Read the model definition and answer for the solid it produces. Units are mm, in the model's axes. A direction names the side the tool comes from. Round coordinates to 2 decimals unless told otherwise and drop trailing zeros. Order: outer loops, then holes, each group sorted by start corner. A loop starts at its lowest first (then second) coordinate and runs counter-clockwise, first axis right, second up. Notation, with made-up numbers: (23.25, 66.5) -> (58.25, 66.5) arc R18 ccw to (58.25, 101.5) -> close; hole circle Ø4 at (49.5, -14). An arc over 180 degrees is marked (long way). Answer as a JSON object with one key per item and string values. Group by question number.
Item 1: Section C-C, the plane z = -9 is taken. Write down the section's boundary in (x, y), plus the area to 3 significant figures.
Item 2: For faces 1 (the cylindrical face through (22.15, 22.6, -13.87)), 2 (the flat face through (-1, 15, 8.899)), determine the directions among +Z, -Z, +X, -X, +Y, -Y from which every point of the face is accessible in a straight line to the end or side of a thin tool.
Item 3: The mould has two halves that part along X. Classify faces 3 (the flat face through (40, 15, -11)), 4 (the cylindrical face through (-22.15, 22.6, -8.33)), 5 (the flat face through (-1, 30, -11)): pulls with the +X half, pulls with the -X half, needs draft (parallel to the pull), parting line crosses it, or undercut.
Item 4: Section B-B, the plane y = 12.5 is taken. Write down the section's boundary in (x, z), plus the area to 3 significant figures.
Item 5: Section A-A, the plane x = -33 is taken. Write down the section's boundary in (y, z), plus the area to 3 significant figures.
Item 6: Consider probe 1 along X at (y, z) = (19.75, -13.5); probe 2 along X at (y, z) = (20.75, -8.5); probe 3 along Z at (x, y) = (-23, 28.25). Determine where each line is inside the solid, lowest interval first. Write a range as from..to.
Item 7: Section D-D, the plane y = 19 is taken. Write down the section's boundary in (x, z), plus the area to 3 significant figures.
from build123d import *

# Parameters (mm, degrees)
SKETCH1_W           = 80
SKETCH1_H           = 40
SKETCH1_R           = 3
BOSS_EXTRUDE1_DEPTH = 30
SKETCH2_R           = 3
CUT_EXTRUDE1_DEPTH  = 15


with BuildPart() as part:
    # Sketch1 → Boss-Extrude1 (new body)
    with BuildSketch(Plane(origin=(0, 0, 0), x_dir=(1, 0, 0), z_dir=(0, 1, 0))):
        with Locations((0, 11.100547393)):
            Rectangle(SKETCH1_W, SKETCH1_H)
        with Locations(Location((-33, 11.100547393, 0), (0, 0, 270))):  # turned: the seam where the file's is
            Circle(SKETCH1_R, mode=Mode.SUBTRACT)
        with Locations(Location((33, 11.100547393, 0), (0, 0, 90))):  # turned: the seam where the file's is
            Circle(SKETCH1_R, mode=Mode.SUBTRACT)
    extrude(amount=BOSS_EXTRUDE1_DEPTH)

    # Sketch2 → Cut-Extrude1 (cut)
    with BuildSketch(Plane(origin=(0, 30, 0), x_dir=(-1, 0, 0), z_dir=(0, 1, 0))):
        with Locations(Location((21, -11.100547393, 0), (0, 0, 90))):  # turned: the seam where the file's is
            Circle(SKETCH2_R)
        with Locations(Location((-21, -11.100547393, 0), (0, 0, 270))):  # turned: the seam where the file's is
            Circle(SKETCH2_R)
    extrude(amount=-CUT_EXTRUDE1_DEPTH, mode=Mode.SUBTRACT)


solid = part.part
Values found:
{
 "1": {"outline": "(-40, 0) -> (-35.14, 0) -> (-35.14, 30) -> (-40, 30) -> close; (-30.86, 0) -> (30.86, 0) -> (30.86, 30) -> (23.14, 30) -> (23.14, 15) -> (18.86, 15) -> (18.86, 30) -> (-18.86, 30) -> (-18.86, 15) -> (-23.14, 15) -> (-23.14, 30) -> (-30.86, 30) -> close; (35.14, 0) -> (40, 0) -> (40, 30) -> (35.14, 30) -> close", "area": "2,010 mm2"},
 "2": {"face 1": "+Y", "face 2": "+Z, +X, -X, +Y, -Y"},
 "3": {"face 3": "pulls with the +X half", "face 4": "undercut", "face 5": "needs draft"},
 "4": {"outline": "(-40, -31.1) -> (40, -31.1) -> (40, 8.9) -> (-40, 8.9) -> close; hole circle Ø6 at (-33, -11.1); hole circle Ø6 at (33, -11.1)", "area": "3,140 mm2"},
 "5": {"outline": "(0, -31.1) -> (30, -31.1) -> (30, -14.1) -> (0, -14.1) -> close; (0, -8.1) -> (30, -8.1) -> (30, 8.9) -> (0, 8.9) -> close", "area": "1,020 mm2"},
 "6": {"probe 1": "-40..-34.8, -31.2..-22.8, -19.2..19.2, 22.8..31.2, 34.8..40", "probe 2": "-40..-34.5, -31.5..-22.5, -19.5..19.5, 22.5..31.5, 34.5..40", "probe 3": "-31.1..-13.34, -8.86..8.9"},
 "7": {"outline": "(-40, -31.1) -> (40, -31.1) -> (40, 8.9) -> (-40, 8.9) -> close; hole circle Ø6 at (-33, -11.1); hole circle Ø6 at (-21, -11.1); hole circle Ø6 at (21, -11.1); hole circle Ø6 at (33, -11.1)", "area": "3,090 mm2"}
}
